Here's how the part is built. I have some questions about the finished solid (model axes, mm). A direction names the side the tool comes from. Round coordinates to 2 decimals unless told otherwise and drop trailing zeros. Write each loop counter-clockwise with the first axis right and the second up, starting at its lowest first coordinate (ties: lowest second). Pieces come first, ordered by that corner, then holes. Notation, with made-up numbers: (85, -32) -> (93, -32) arc R14 ccw to (93, -23) -> close; hole circle Ø2 at (42, 16). An arc over 180 degrees is marked (long way). Put each result on its own line as item: value. Start each with the question number.
1. Which directions (+Z, -Z, +X, -X, +Y, -Y) give clear straight access to the entire face, cutting with the end or side of a thin tool? Please do faces 5 (the face through (15.7, 0.95, 11.79)), 6 (the face through (68.945, 19.317, 2.22)), 7 (the face through (41.44, 3.131, 46.683)), 8 (the face through (68.9, 0.91, 27.14)), 9 (the face through (68.94, 11.75, 27.14)).
2. Suppose I cut it at D-D (z = 22.5). Please give me the cut outline in (x, y) (3 decimals).
3. Suppose I cut it at B-B (x = 50.8). Please give me the cut outline in (y, z) (3 decimals).
4. We'd pull the mould along Z, two halves only. Please class faces 1 (the face through (32.705, 19.317, 2.27)), 2 (the face through (100.65, 18.83, 11.79)), 3 (the face through (51, 12.7, 31)), 4 (the face through (56.747, 9.569, 38.362)): +Z half, -Z half, draft (parallel to the pull), parting line (faces both ways), or undercut.
5. Suppose I cut it at A-A (y = 25.4). Count the separate pieces of the cut face and the enclosed holes in it, then the cut area to 3 significant figures.
6. I need wall thicknesses on probe 1 along Z at (x, y) = (50.8, 9.5) (3 decimals); probe 2 along Y at (x, z) = (12.7, 7.5); probe 3 along X at (y, z) = (8.5, 38.5). Which ranges of each line are inside material? Lowest first, please. Write a range as from..to.
7. For pin 1 (5 mm diameter, centred on y = 5.5, z = 32, fed in from +X); pin 2 (10 mm diameter, centred on x = 39, z = 47.5, fed in from -Y); pin 3 (16 mm diameter, centred on x = 65.5, y = 17, fed in from +Z); pin 4 (7.5 mm diameter, centred on x = 56, z = 37, fed in from -Y), each with a flat end and sliding along its axis, tell me the tip position at first contact or that it passes through.
```python
from build123d import *

# Parameters (mm, degrees)
F0_W           = 101.6
F0_H           = 38.1
F1_DEPTH       = 12.7
F3_DEPTH       = 12.7
F5_D           = 11.90625
F5_CBORE_D     = 25.4
F5_CBORE_DEPTH = 6.35
F6_W           = 38.1
F6_H           = 3.175
F7_DEPTH       = 38.101
F9_D           = 10.0838
F10_R          = 3.17499
F11_R          = 3.17499


# Not quite as in the source:
# - a fillet or chamfer is up to 0.001 mm smaller than in the source, because OpenCascade refuses the exact size
# - a length typed as a fraction of an inch, garbled in the dataset ("3 / 203.2 mm" for 3/8 in), is restored


with BuildPart() as f1:
    # F0 (on Top) → F1 (new body)
    with BuildSketch(Plane.XY):
        with Locations((50.8, 19.05)):
            Rectangle(F0_W, F0_H)
    extrude(amount=F1_DEPTH)

    # F2 (on Front) → F3 (join)
    with BuildSketch(Plane.XZ):
        with BuildLine():
            Line((31.75, 38.1), (31.75, 0))
            Line((31.75, 0), (69.85, 0))
            Line((69.85, 0), (69.85, 38.1))
            ThreePointArc((69.85, 38.1), (50.8, 57.15), (31.75, 38.1))
        make_face()
    extrude(amount=-F3_DEPTH)

    # F5 (through all)
    with Locations(Plane.XZ):
        with Locations((50.8, 38.1)):
            CounterBoreHole(F5_D / 2, F5_CBORE_D / 2, F5_CBORE_DEPTH)

    # F6 (on face) → F7 (cut, through all)
    with BuildSketch(Plane.XZ):
        with Locations((50.8, 1.5875)):
            Rectangle(F6_W, F6_H)
    extrude(amount=-F7_DEPTH, mode=Mode.SUBTRACT)

    # F9 (through all)
    with Locations(Plane.XY.offset(12.7)):
        with Locations((12.7, 25.4), (88.9, 25.4)):
            Hole(F9_D / 2)

    # F10 (radius 3.175 in the source; OpenCascade refuses exactly that, so slightly less here)
    f10_edges = [f1.edges().sort_by_distance(p)[0] for p in [
        (0, 0, 6.35),
        (0, 38.1, 6.35),
        (101.6, 0, 6.35),
        (101.6, 38.1, 6.35),
        (31.75, 19.05, 3.175),
        (69.85, 19.05, 3.175),
    ]]
    fillet(f10_edges, radius=F10_R)

    # F11 (radius 3.175 in the source; OpenCascade refuses exactly that, so slightly less here)
    f11_edges = [f1.edges().sort_by_distance(p)[0] for p in [
        (50.8, 38.1, 12.7),
        (101.6, 19.05, 12.7),
        (100.670067, 37.170067, 12.7),
        (100.670067, 0.929933, 12.7),
        (84.137505, 0, 12.7),
        (0.929933, 37.170067, 12.7),
        (0, 19.05, 12.7),
        (0.929933, 0.929933, 12.7),
        (17.462495, 0, 12.7),
        (31.75, 0, 25.4),
        (50.8, 0, 57.15),
        (69.85, 0, 25.4),
        (69.85, 6.35, 12.7),
        (31.75, 6.35, 12.7),
        (50.8, 12.7, 12.7),
        (31.75, 12.7, 25.4),
        (50.8, 12.7, 57.15),
        (69.85, 12.7, 25.4),
    ]]
    fillet(f11_edges, radius=F11_R)


solid = f1.part
```
Verdict:
1. face 5: +Z, -X, -Y
1. face 6: -Z, +Y, -Y
1. face 7: -Y
1. face 8: +Z, +X, -Y
1. face 9: +Z, +X, +Y
2. outline: (31.75, 3.175) arc R3.175 ccw to (34.925, 0) -> (66.675, 0) arc R3.175 ccw to (69.85, 3.175) -> (69.85, 9.525) arc R3.175 ccw to (66.675, 12.7) -> (34.925, 12.7) arc R3.175 ccw to (31.75, 9.525) -> close
3. outline: (0, 3.175) -> (38.1, 3.175) -> (38.1, 9.525) arc R3.175 ccw to (34.925, 12.7) -> (15.875, 12.7) arc R3.175 cw to (12.7, 15.875) -> (12.7, 32.147) -> (6.35, 32.147) -> (6.35, 25.4) -> (0, 25.4) -> close; (0, 50.8) -> (6.35, 50.8) -> (6.35, 44.053) -> (12.7, 44.053) -> (12.7, 53.975) arc R3.175 ccw to (9.525, 57.15) -> (3.175, 57.15) arc R3.175 ccw to (0, 53.975) -> close
4. face 1: -Z half
4. face 2: +Z half
4. face 3: draft
4. face 4: undercut
5. separate pieces: 3
5. enclosed holes: 0
5. area: 913 mm^2
6. probe 1: z = 3.175..32.147, 44.053..57.15
6. probe 2: y = 0..20.36, 30.44..38.1
6. probe 3: x = 31.75..44.86, 56.74..69.85
7. pin 1: stops at x = 69.85
7. pin 2: stops at y = 0
7. pin 3: stops at z = 54.25
7. pin 4: stops at y = 6.35
